Drawing for the job (mm, zero at the part's lowest x, y, z). A direction names the side the tool comes from. Coordinates: 2 decimals unless noted, no trailing zeros. Loops run counter-clockwise (first coordinate to the right, second up) from the corner with the lowest first, then second, coordinate; pieces in that order, holes last. Notation, with made-up numbers: (24, 26) - (38, 26) arc R27 cw to (38, 44) - close; hole circle Ø2 at (-24.5, -13.75). An arc over 180 degrees is marked (long way). One line per item, written item: value.
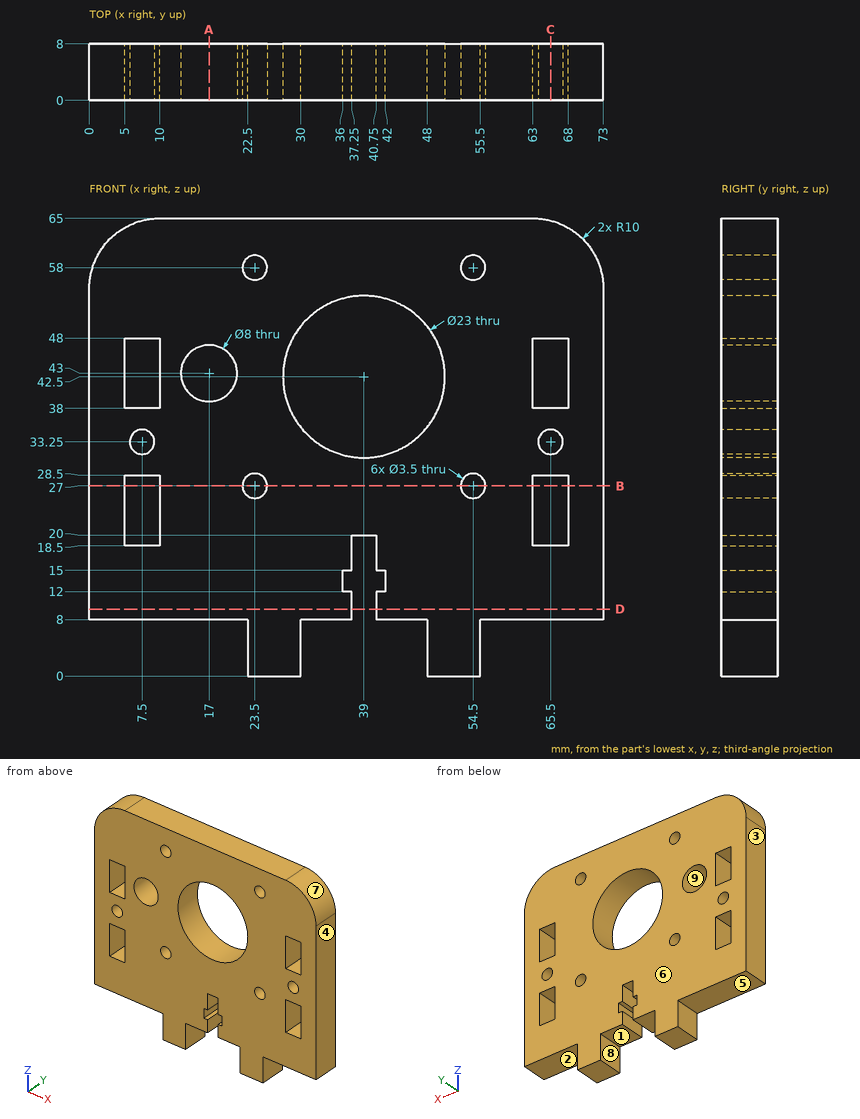
Item 1: Cut at B-B, the plane z = 27. Write the cut outline in (x, y).
Check result:
outline: (0, 0) - (5, 0) - (5, 8) - (0, 8) - close; (10, 0) - (21.75, 0) - (21.75, 8) - (10, 8) - close; (25.25, 0) - (52.75, 0) - (52.75, 8) - (25.25, 8) - close; (56.25, 0) - (63, 0) - (63, 8) - (56.25, 8) - close; (68, 0) - (73, 0) - (73, 8) - (68, 8) - close
Item 2: Pull direction X, two halves, no side cores. Call the marked faces 6, 7, 8 and 9: released by +X, released by -X, zero draft, split by the parting line, or undercut.
Check result:
face 6: zero draft
face 7: released by +X
face 8: undercut
face 9: undercut
Item 3: Tool access for the marked faces 1, 2, 3, 4 and 5: list every direction of +Z, -Z, +X, -X, +Y, -Y with a clear straight run to the whole face (end or side of a thin tool).
Check result:
face 1: -Z, +Y, -Y
face 2: -Z, +X, +Y, -Y
face 3: +Z, -Z, -X, +Y, -Y
face 4: +Z, -Z, +X, +Y, -Y
face 5: -Z, -X, +Y, -Y
Item 4: Cut at D-D, the plane z = 9.5. Write the cut outline in (x, y), then the cut area to 3 significant figures.
Check result:
outline: (0, 0) - (37.25, 0) - (37.25, 8) - (0, 8) - close; (40.75, 0) - (73, 0) - (73, 8) - (40.75, 8) - close
area: 556 mm^2
Item 5: Probe probe 1 along X at (y, z) = (3.5, 27); probe 2 along Z at (x, y) = (54.5, 2); probe 3 along X at (y, z) = (4.5, 43). List the from-to ranges inside material, lowest first. Write a range as from..to.
Check result:
probe 1: x = 0..5, 10..21.75, 25.25..52.75, 56.25..63, 68..73
probe 2: z = 0..25.25, 28.75..56.25, 59.75..65
probe 3: x = 0..5, 10..13, 21..27.51, 50.49..63, 68..73
Item 6: Drop flat-ended pins along their axis: P1, Ø1.4, axis at x = 37, y = 5.5, coming from the -Z side; P2, Ø2.5, axis at y = 4, z = 2.5, coming from the -X side; P3, Ø1.5, axis at x = 8, y = 6, coming from the +Z side. Give the stop position or say it passes through.
Check result:
P1: stops at z = 8
P2: stops at x = 22.5
P3: stops at z = 64.92
Item 7: Cut at C-C, the plane x = 65.5. Write the cut outline in (y, z), then the cut area to 3 significant figures.
Check result:
outline: (0, 8) - (8, 8) - (8, 18.5) - (0, 18.5) - close; (0, 28.5) - (8, 28.5) - (8, 31.5) - (0, 31.5) - close; (0, 35) - (8, 35) - (8, 38) - (0, 38) - close; (0, 48) - (8, 48) - (8, 64.68) - (0, 64.68) - close
area: 265 mm^2
Item 8: Cut at A-A, the plane x = 17. Write the cut outline in (y, z), then the cut area to 3 significant figures.
Check result:
outline: (0, 8) - (8, 8) - (8, 39) - (0, 39) - close; (0, 47) - (8, 47) - (8, 65) - (0, 65) - close
area: 392 mm^2
